Geometry check sheet. Reference: the model listing, model coordinates, mm. Coordinates: 2 decimals unless noted, no trailing zeros. Order: outer loops, then holes, each group sorted by start corner. A loop starts at its lowest first (then second) coordinate and runs counter-clockwise, first axis right, second up. Notation, with made-up numbers: M 22.5,81 L 50.5,81 A21 ccw 50.5,99 Z; hole C 19.25,57 d5. An arc over 180 degrees is marked long. Use CSV: the item, a comma, the result in double quotes. Start each with the question number.
```python
from build123d import *

# Parameters (mm, degrees)
F0_R     = 13.2
F0_W     = 1.5
F0_H     = 3.5
F1_DEPTH = 2.8


with BuildPart() as f1:
    # F0 (on Top) → F1 (new body)
    with BuildSketch(Plane.XY):
        Circle(F0_R)
        Polygon((-5.765517, -9.631268), (-6.998184, -8.776555), (-5.003855, -5.900333), (-3.771189, -6.755045), align=None, mode=Mode.SUBTRACT)
        Polygon((-2.527204, -10.936898), (-3.962865, -10.502295), (-2.948791, -7.152421), (-1.513131, -7.587024), align=None, mode=Mode.SUBTRACT)
        Polygon((-8.445988, -7.393766), (-9.356395, -6.201643), (-6.574773, -4.07736), (-5.664366, -5.269484), align=None, mode=Mode.SUBTRACT)
        Polygon((-10.30927, -4.440883), (-10.809331, -3.026691), (-7.50955, -1.859883), (-7.009489, -3.274075), align=None, mode=Mode.SUBTRACT)
        Polygon((-11.175082, -1.058324), (-11.216413, 0.441107), (-7.717742, 0.537547), (-7.676411, -0.961884), align=None, mode=Mode.SUBTRACT)
        Polygon((0.955627, -11.184332), (-0.54412, -11.211888), (-0.608418, -7.712479), (0.891329, -7.684922), align=None, mode=Mode.SUBTRACT)
        Polygon((4.345997, -10.349629), (2.927271, -10.836678), (1.790823, -7.526317), (3.209549, -7.039268), align=None, mode=Mode.SUBTRACT)
        Polygon((7.315871, -8.51355), (6.115435, -9.412968), (4.016793, -6.611949), (5.21723, -5.712531), align=None, mode=Mode.SUBTRACT)
        Polygon((9.5779, -5.853745), (8.711901, -7.078508), (5.85412, -5.057844), (6.720119, -3.83308), align=None, mode=Mode.SUBTRACT)
        Polygon((10.913222, -2.627562), (10.46545, -4.05917), (7.125032, -3.014368), (7.572805, -1.58276), align=None, mode=Mode.SUBTRACT)
        Polygon((-10.959651, 2.426634), (-10.538254, 3.866225), (-7.179207, 2.882966), (-7.600603, 1.443374), align=None, mode=Mode.SUBTRACT)
        Polygon((-9.683822, 5.676803), (-8.840469, 6.917269), (-5.946049, 4.949445), (-6.789402, 3.708979), align=None, mode=Mode.SUBTRACT)
        Polygon((-7.471038, 8.377714), (-6.287327, 9.299033), (-4.137583, 6.537041), (-5.321293, 5.615722), align=None, mode=Mode.SUBTRACT)
        Polygon((-4.535395, 10.268042), (-3.125856, 10.781072), (-1.928786, 7.492148), (-3.338325, 6.979118), align=None, mode=Mode.SUBTRACT)
        with BuildLine():
            ThreePointArc((1.5, 2), (2.236068, 1.118034), (2.5, 0))
            ThreePointArc((2.5, 0), (2.236068, -1.118034), (1.5, -2))
            ThreePointArc((1.5, -2), (0, -2.5), (-1.5, -2))
            ThreePointArc((-1.5, -2), (-2.5, 0), (-1.5, 2))
            ThreePointArc((-1.5, 2), (0, 2.5), (1.5, 2))
        make_face(mode=Mode.SUBTRACT)
        Polygon((11.192638, 0.852849), (11.206417, -0.647087), (7.706564, -0.679238), (7.692786, 0.820699), align=None, mode=Mode.SUBTRACT)
        Polygon((10.389113, 4.250744), (10.86311, 2.827604), (7.54245, 1.721612), (7.068453, 3.144752), align=None, mode=Mode.SUBTRACT)
        Polygon((8.580393, 7.237359), (9.468746, 6.028711), (6.648568, 3.955888), (5.760215, 5.164535), align=None, mode=Mode.SUBTRACT)
        with Locations((0, 9.45)):
            Rectangle(F0_W, F0_H, mode=Mode.SUBTRACT)
        Polygon((2.727698, 10.888625), (4.155132, 10.427722), (3.07969, 7.097042), (1.652256, 7.557946), align=None, mode=Mode.SUBTRACT)
        Polygon((5.941479, 9.523725), (7.158235, 8.646512), (5.111405, 5.807412), (3.894648, 6.684625), align=None, mode=Mode.SUBTRACT)
        with BuildLine():
            Line((-1.5, -2), (-1.5, 2))
            ThreePointArc((-1.5, 2), (-2.5, 0), (-1.5, -2))
        make_face()
        with BuildLine():
            ThreePointArc((1.5, -2), (2.236068, -1.118034), (2.5, 0))
            ThreePointArc((2.5, 0), (2.236068, 1.118034), (1.5, 2))
            Line((1.5, 2), (1.5, -2))
        make_face()
    extrude(amount=F1_DEPTH)


solid = f1.part
```
1) Draft check along Y on faces 1 (the face through (0.75, 9, 1)), 2 (the face through (-7.414, 5.947, 1.38)). Enter one of: +Y half, -Y half, draft (parallel to the pull), parting line (faces both ways), or undercut.
2) Material ranges on line 1 along Y through (x, z) = (8.25, 1.3); line 2 along Y through (x, z) = (6.5, 0.75); line 3 along Y through (x, z) = (-9.5, 0.75), recorded low to high.
3) Section check B-B on x = 0. Record the boundary of the cut face in (y, z), then the cut area to 3 significant figures.
4) Gauge pin test, flat ends, axial feed: P1, Ø1.4, axis at y = 9, z = 0.5, coming from the -X side; P2, Ø0.8, axis at y = 9.5, z = 1, coming from the +X side. Record the tip position at first contact, or that the pin passes through.
5) Section check A-A on y = 0. Record the boundary of the cut face in (x, z), then the cut area to 3 significant figures.
6) Section check C-C on z = 0.35. State how many separate pieces and enclosed holes the cut face has, then the cut area to 3 significant figures.
Results are:
1,face 1,"undercut"
1,face 2,"undercut"
2,line 1,"y = -10.3 to -6.75, -4.91 to -3.37, -1.79 to -0.67, 0.83 to 1.96, 3.54 to 5.13, 6.99 to 10.3"
2,line 2,"y = -11.49 to -9.12, -7.42 to -5.51, -4.14 to 4.16, 5.71 to 7.73, 9.12 to 11.49"
2,line 3,"y = -9.16 to -4.15, -2.56 to -1.01, 0.49 to 2, 3.56 to 5.55, 5.95 to 9.16"
3,outline,"M -13.2,0 L -11.2,0 L -11.2,2.8 L -13.2,2.8 Z; M -7.7,0 L -2.5,0 L -2.5,2.8 L -7.7,2.8 Z; M 2.5,0 L 7.7,0 L 7.7,2.8 L 2.5,2.8 Z; M 11.2,0 L 13.2,0 L 13.2,2.8 L 11.2,2.8 Z"
3,area,"40.3 mm²"
4,P1,"stops at x = -10.26"
4,P2,"stops at x = 9.56"
5,outline,"M -13.2,0 L -11.2,0 L -11.2,2.8 L -13.2,2.8 Z; M -7.7,0 L -1.5,0 L -1.5,2.8 L -7.7,2.8 Z; M 1.5,0 L 7.7,0 L 7.7,2.8 L 1.5,2.8 Z; M 11.2,0 L 13.2,0 L 13.2,2.8 L 11.2,2.8 Z"
5,area,"45.9 mm²"
6,separate pieces,"1"
6,enclosed holes,"21"
6,area,"428 mm²"
